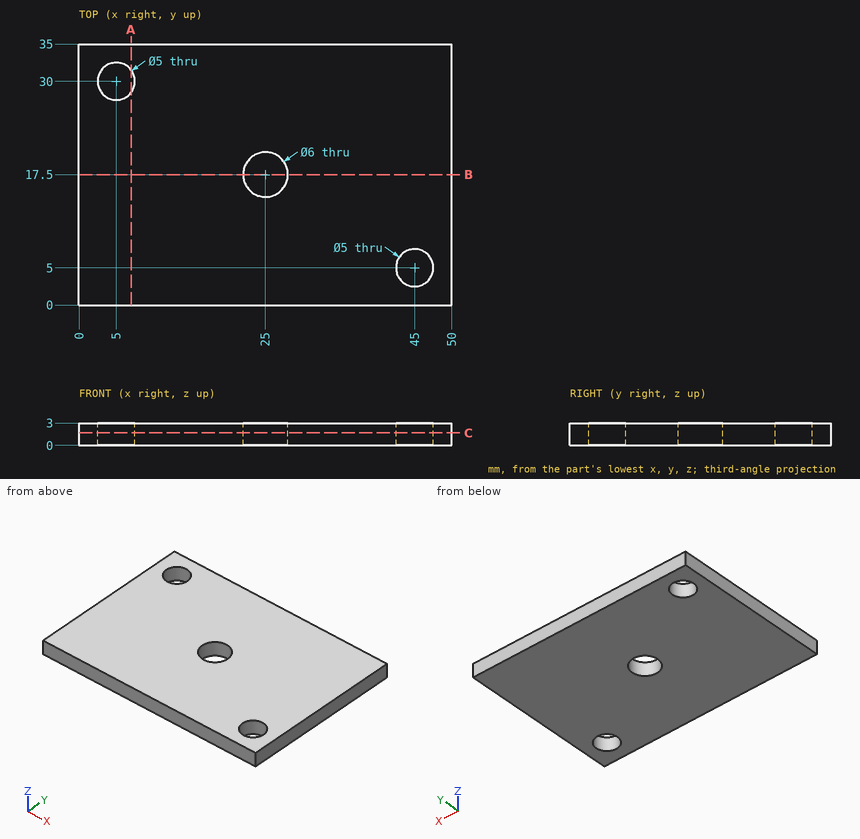
Design review of the part shown in the three views and the two pictorial views. Dimensions are in mm from the part's minimum x, y and z. Give positions to 0.01 mm unless a question says otherwise; leave off trailing zeros. Order: outer loops, then holes, each group sorted by start corner. A loop starts at its lowest first (then second) coordinate and runs counter-clockwise, first axis right, second up. Notation, with made-up numbers: M 46.5,12.25 L 73.5,12.25 A24 ccw 73.5,47.25 Z; hole C 9.25,73 d11. An arc over 180 degrees is marked long. Answer in a Markdown table with one row per item. Add a question column.
(1) Consider section A-A on x = 7. State the section outline as (y, z) points.
(2) Wall thickness on probe 1 along Y at (x, z) = (25, 2.35); probe 2 along X at (y, z) = (30, 0.7); probe 3 along X at (y, z) = (5, 1.95): over which ranges is each line inside the solid? List them lowest first. Write a range as [from, to].
(3) For pin 1 (5 mm diameter, centred on x = 25, y = 17.5, fed in from +Z); pin 2 (2 mm diameter, centred on x = 10, y = 26.5, fed in from -Z), all flat-tipped, find the tip position at first contact; note any pin that passes through.
(4) Consider section B-B on y = 17.5. State the section outline as (x, z) points.
(5) Consider section C-C on z = 1.7. State the section outline as (x, y) points.
Evaluation:
| question | item | result |
|---|---|---|
| 1 | outline | M 0,0 L 28.5,0 L 28.5,3 L 0,3 Z; M 31.5,0 L 35,0 L 35,3 L 31.5,3 Z |
| 2 | probe 1 | y = [0, 14.5], [20.5, 35] |
| 2 | probe 2 | x = [0, 2.5], [7.5, 50] |
| 2 | probe 3 | x = [0, 42.5], [47.5, 50] |
| 3 | pin 1 | passes through |
| 3 | pin 2 | stops at z = 0 |
| 4 | outline | M 0,0 L 22,0 L 22,3 L 0,3 Z; M 28,0 L 50,0 L 50,3 L 28,3 Z |
| 5 | outline | M 0,0 L 50,0 L 50,35 L 0,35 Z; hole C 5,30 d5; hole C 25,17.5 d6; hole C 45,5 d5 |
